Read the model definition and answer for the solid it produces. Units are mm, in the model's axes. Face numbers are marked on the shaded views. Coordinates: 2 decimals unless noted, no trailing zeros. Order: outer loops, then holes, each group sorted by start corner. A loop starts at its lowest first (then second) coordinate and runs counter-clockwise, first axis right, second up. Notation, with made-up numbers: (-1.75, 39) -> (9.25, 39) arc R17 cw to (9.25, 57) -> close; hole circle Ø6 at (23.25, -9.5). An arc over 180 degrees is marked (long way). Answer in a Markdown table with one row per item.
from build123d import *

# Parameters (mm, degrees)
PAD008_DEPTH    = 10.75
SKETCH049_W     = 19.5
SKETCH049_H     = 9.508905554
POCKET006_DEPTH = 6.8868250221
POCKET007_DEPTH = 1


with BuildPart() as part:
    # Sketch048 → Pad008 (new body, symmetric)
    with BuildSketch(Plane.YZ):
        with BuildLine():
            ThreePointArc((-17.570923429, -35.349067746), (-11.5889977168, -37.5087777423), (-5.3676713633, -36.1885955969))
            ThreePointArc((-4.0896315326, -39.9266740125), (-2.5394656722, -37.309157564), (-5.3676713633, -36.1885955969))
            ThreePointArc((-17.7649340088, -35.5765725595), (-11.4595142974, -39.4247858993), (-4.0896315326, -39.9266740125))
            ThreePointArc((-17.570923429, -35.349067746), (-17.7727328087, -35.3734457702), (-17.7649340088, -35.5765725595))
        make_face()
    extrude(amount=PAD008_DEPTH, both=True)

    # Sketch049 (on DatumPlane) → Pocket006 (cut, through all)
    with BuildSketch(Plane(origin=(10.75, -4.0896315326, -39.9266740125), x_dir=(1, 0, 0), z_dir=(0, 0.1711412337, -0.9852465063))):
        with Locations((-10.75, 5.754452777)):
            Rectangle(SKETCH049_W, SKETCH049_H)
    extrude(amount=-POCKET006_DEPTH, mode=Mode.SUBTRACT)

    # Sketch050 → Pocket007 (cut, symmetric)
    with BuildSketch(Plane.YZ):
        Polygon((-16.49066, -37.494777), (-15.936452, -36.755833), (-13.493837, -38.459507), (-14.520146, -39.301079), align=None)
    extrude(amount=POCKET007_DEPTH, both=True, mode=Mode.SUBTRACT)


solid = part.part
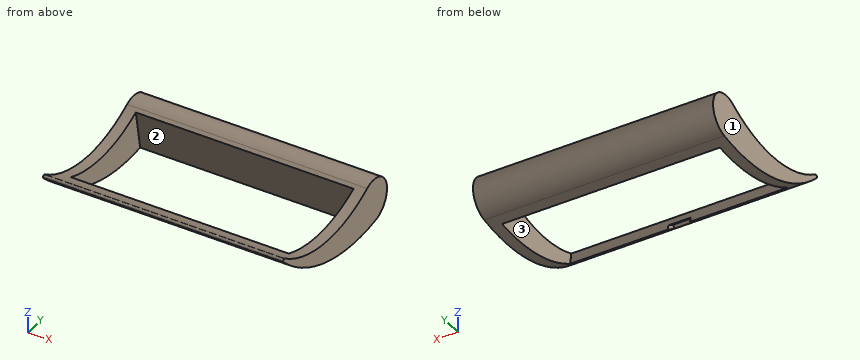
Q1. The part is cut by section B-B (x = 6.25). Write down the section's boundary in (y, z), then the cut area to 3 significant figures.
Outcome:
| item | result |
|---|---|
| outline | (-17.76, -35.58) arc R15.54 ccw to (-15.14, -37.69) -> (-15.33, -36.61) arc R11.6 cw to (-17.57, -35.35) arc R0.15 ccw to start; (-5.72, -36.37) -> (-5.08, -40.07) arc R15.54 ccw to (-4.09, -39.93) arc R2 ccw (long way) to (-5.37, -36.19) arc R11.6 cw to start |
| area | 11.9 mm² |
Q2. For a pull along Y with two mould halves and no side action, classify the marked faces 1, 2 and 3 as pulls with the +Y half, pulls with the -Y half, needs draft (parallel to the pull), parting line crosses it, or undercut.
Outcome:
| item | result |
|---|---|
| face 1 | needs draft |
| face 2 | undercut |
| face 3 | undercut |
Q3. Given pin 1 (1 mm diameter, centred on x = 4.5, z = -38, fed in from -Y); pin 2 (2 mm diameter, centred on y = -8, z = -36.5, fed in from -X); pin 3 (3 mm diameter, centred on x = -6, y = -5, fed in from -Z); pin 4 (1 mm diameter, centred on x = 1.5, z = -37.5, fed in from -Y), each flat-ended and moving along its own axis, determine where each tip first touches the part or whether it passes through.
Outcome:
| item | result |
|---|---|
| pin 1 | y = -15.44 |
| pin 2 | x = -10.75 |
| pin 3 | z = -40.07 |
| pin 4 | y = -16.14 |
Q4. Consider line 1 (X direction, y = -9.5, z = -39.55); line 2 (Y direction, x = 6.5, z = -37.35); line 3 (Y direction, x = -4.75, z = -39.45). Determine where each line is inside the solid, lowest interval first.
Outcome:
| item | result |
|---|---|
| line 1 | -10.75 to -9.75, 9.75 to 10.75 |
| line 2 | -15.66 to -15.2, -5.55 to -2.53 |
| line 3 | -5.19 to -3.1 |
Q5. The part is cut by section C-C (z = -39.15). Write down the section's boundary in (x, y).
Outcome:
| item | result |
|---|---|
| outline | (-10.75, -12.25) -> (-9.75, -12.25) -> (-9.75, -5.24) -> (9.75, -5.24) -> (9.75, -12.25) -> (10.75, -12.25) -> (10.75, -2.83) -> (-10.75, -2.83) -> close |
Q6. The part is cut by section D-D (x = -0.5). Write down the section's boundary in (y, z).
Outcome:
| item | result |
|---|---|
| outline | (-17.76, -35.58) arc R15.54 ccw to (-16.13, -37.01) -> (-15.94, -36.76) -> (-15.22, -37.26) -> (-15.33, -36.61) arc R11.6 cw to (-17.57, -35.35) arc R0.15 ccw to start; (-5.72, -36.37) -> (-5.08, -40.07) arc R15.54 ccw to (-4.09, -39.93) arc R2 ccw (long way) to (-5.37, -36.19) arc R11.6 cw to start |
Q7. The part is cut by section A-A (y = -11.75). Write down the section's boundary in (x, z), then the cut area to 3 significant figures.
Outcome:
| item | result |
|---|---|
| outline | (-10.75, -39.33) -> (-9.75, -39.33) -> (-9.75, -37.5) -> (-10.75, -37.5) -> close; (9.75, -39.33) -> (10.75, -39.33) -> (10.75, -37.5) -> (9.75, -37.5) -> close |
| area | 3.67 mm² |
